Input: part model. Units: mm. Frame: model coordinates. Face numbers are marked on the shaded views. Give positions to 0.01 mm unless a question says otherwise; leave off trailing zeros. Write each loop counter-clockwise with the first axis right and the second up, starting at its lowest first coordinate (ties: lowest second). Pieces come first, ordered by that corner, then holes. Notation, with made-up numbers: (-17, 31) - (27, 31) arc R21 ccw to (27, 51) - close; hole circle Ø8 at (61.25, 3.25). An arc over 180 degrees is marked (long way). Answer as a JSON object with one key per item and string values. Group by question number.
from build123d import *

# Parameters (mm, degrees)
F2_R           = 0.5
F3_SIZE2       = 0.1154700538
F3_SIZE        = 0.2
F3_2_SIZE2     = 0.1154700538
F3_2_SIZE      = 0.2
F6_D           = 1.2
F6_DEPTH       = 2
F6_TIP         = 0.3605163714
F7_D           = 1
F7_DEPTH       = 2.2
F7_CSINK_D     = 2
F7_CSINK_ANGLE = 60
F7_TIP         = 0.3004303095
F8_D           = 2
F8_DEPTH       = 8.5
F8_CBORE_D     = 2.5
F8_CBORE_DEPTH = 1.5
F8_TIP         = 0.600860619


with BuildPart() as f1:
    # F0 (on Front) → F1 (revolve)
    with BuildSketch(Plane.XZ):
        with BuildLine():
            Line((0, 4.5), (0, 0))
            Line((0, 0), (27.05, 0))
            Line((27.05, 0), (27.05, 2.49625))
            Line((27.05, 2.49625), (19.825, 2.49625))
            Line((19.825, 2.49625), (18.9654697867, 2))
            Line((18.9654697867, 2), (9.6845302133, 2))
            Line((9.6845302133, 2), (8.825, 2.49625))
            Line((8.825, 2.49625), (4.302, 2.49625))
            Line((4.302, 2.49625), (4.1752050808, 2.4230449192))
            ThreePointArc((4.1752050808, 2.4230449192), (4.1269688898, 2.4030648347), (4.0752050808, 2.39625))
            Line((4.0752050808, 2.39625), (4.025, 2.39625))
            ThreePointArc((4.025, 2.39625), (3.8835786438, 2.4548286438), (3.825, 2.59625))
            Line((3.825, 2.59625), (3.825, 3.74825))
            Line((3.825, 3.74825), (1.202, 3.74825))
            Line((1.202, 3.74825), (1.0752050808, 3.6750449192))
            ThreePointArc((1.0752050808, 3.6750449192), (1.0269688898, 3.6550648347), (0.9752050808, 3.64825))
            Line((0.9752050808, 3.64825), (0.925, 3.64825))
            ThreePointArc((0.925, 3.64825), (0.7835786438, 3.7068286438), (0.725, 3.84825))
            Line((0.725, 3.84825), (0.725, 4.5))
            Line((0.725, 4.5), (0, 4.5))
        make_face()
    revolve(axis=Axis((13.525, 0, 0), (-1, 0, 0)))

    # F2
    f2_edges = [f1.edges().sort_by_distance(p)[0] for p in [
        (9.68453, 0, -2),
        (18.96547, 0, -2),
    ]]
    fillet(f2_edges, radius=F2_R)

    # F3
    f3_edges = [f1.edges().sort_by_distance(p)[0] for p in [
        (27.05, 0, -2.49625),
    ]]
    f3_side = f1.faces().sort_by_distance((23.4375, 0, -2.49625))[0]
    chamfer(f3_edges, length=F3_SIZE, length2=F3_SIZE2, reference=f3_side)

    # F3#2
    f3_2_edges = [f1.edges().sort_by_distance(p)[0] for p in [
        (3.825, 0, -3.74825),
    ]]
    f3_2_side = f1.faces().sort_by_distance((2.5135, 0, -3.74825))[0]
    chamfer(f3_2_edges, length=F3_2_SIZE, length2=F3_2_SIZE2, reference=f3_2_side)

    # F6
    with Locations(Plane(origin=(0, 0, 0), x_dir=(0, -1, 0), z_dir=(-1, 0, 0))):
        with Locations((0, 2), (0, -2)):
            Hole(F6_D / 2, depth=F6_DEPTH)
            with Locations((0, 0, -(F6_DEPTH + F6_TIP / 2))):  # 118° drill point
                Cone(0, F6_D / 2, F6_TIP, mode=Mode.SUBTRACT)

    # F7
    with Locations(Plane(origin=(0, 0, 0), x_dir=(0, -1, 0), z_dir=(-1, 0, 0))):
        with Locations((0, 0)):
            CounterSinkHole(F7_D / 2, F7_CSINK_D / 2, depth=F7_DEPTH, counter_sink_angle=F7_CSINK_ANGLE)
            with Locations((0, 0, -(F7_DEPTH + F7_TIP / 2))):  # 118° drill point
                Cone(0, F7_D / 2, F7_TIP, mode=Mode.SUBTRACT)

    # F8
    with Locations(Plane.YZ.offset(27.05)):
        with Locations((0, 0)):
            CounterBoreHole(F8_D / 2, F8_CBORE_D / 2, F8_CBORE_DEPTH, depth=F8_DEPTH)
            with Locations((0, 0, -(F8_DEPTH + F8_TIP / 2))):  # 118° drill point
                Cone(0, F8_D / 2, F8_TIP, mode=Mode.SUBTRACT)


solid = f1.part
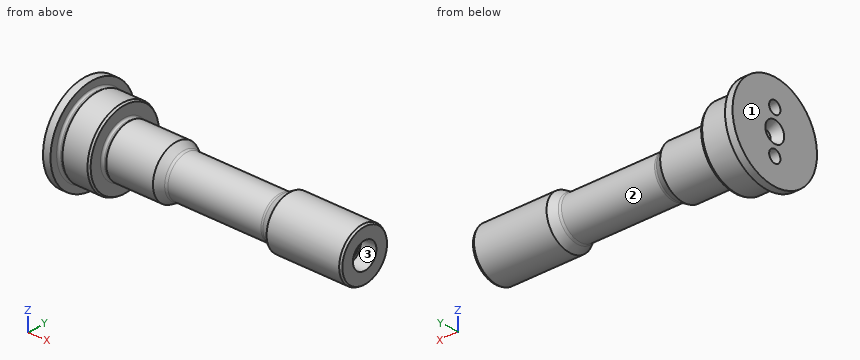
1) Cut plane C-C on x = 12.25. Return the cut outline in (y, z), and give its area (3 significant figures).
2) Cut plane A-A on x = 20.25. Return the cut outline in (y, z).
3) Mould query, pull axis X, two halves, no side actions, for the marked faces 1, 2 and 3. Classes: +X half, -X half, draft (parallel to the pull), parting line (faces both ways), or undercut.
4) Line query: line 1 along Y through (x, z) = (20.5, 0); line 2 along Y through (x, z) = (5.25, -1.5); line 3 along X through (y, z) = (-1.75, 3) (3 decimals). Output: solid intervals per line, ascending. Write a range as from..to.
5) Pin query (flat end, axial travel): P1, Ø3, axis at x = 22, y = 3.5, coming from the -Z side; P2, Ø5, axis at x = 7, z = -1.5, coming from the +Y side; P3, Ø5, axis at x = 6, y = -2, coming from the +Z side. Return the tip coordinate at first contact, or that it passes through.
6) Cut plane B-B on x = 7.75. Return the cut outline in (y, z), and give its area (3 significant figures).
Filled in:
{
 "1": {"outline": "circle Ø4 at (0, 0)", "area": "12.6 mm²"},
 "2": {"outline": "circle Ø4.99 at (0, 0); hole circle Ø2 at (0, 0)"},
 "3": {"face 1": "-X half", "face 2": "undercut", "face 3": "draft"},
 "4": {"line 1": "y = -2.5..-1, 1..2.5", "line 2": "y = -2..2", "line 3": "x = 0..3.825"},
 "5": {"P1": "stops at z = -1.49", "P2": "stops at y = 2.5", "P3": "stops at z = 3.56"},
 "6": {"outline": "circle Ø4.99 at (0, 0)", "area": "19.6 mm²"}
}
